Read the model definition and answer for the solid it produces. Units are mm, in the model's axes. Face numbers are marked on the shaded views. A direction names the side the tool comes from. Coordinates: 2 decimals unless noted, no trailing zeros. Write each loop counter-clockwise with the first axis right and the second up, starting at its lowest first coordinate (ties: lowest second). Pieces come first, ordered by that corner, then holes.
(1) The mould has two halves that part along Z. Classify the marked faces 4, 5 and 6: +Z half, -Z half, draft (parallel to the pull), parting line (faces both ways), or undercut.
(2) Section A-A on x = 36 is taken. Write down the section's boundary in (y, z), then the cut area to 3 significant figures.
(3) Find the intervals of material crossed by probe 1 along Z at (x, y) = (-65.5, -1); probe 2 along Z at (x, y) = (50, -6.5); probe 3 along Z at (x, y) = (19.5, 4.5), in increasing order.
(4) Which of the six approach directions +Z, -Z, +X, -X, +Y, -Y give full straight-line access (tool end or side, diameter ignored) to the marked faces 1, 2 and 3?
(5) Section B-B on y = 5.5 is taken. Write down the section's boundary in (x, z) (3 decimals), then the cut area to 3 significant figures.
(6) Section D-D on y = 32.5 is taken. Write down the section's boundary in (x, z), then the cut area to 3 significant figures.
(7) Section C-C on z = 0 is taken. Write down the section's boundary in (x, y) (3 decimals).
(8) Given pin 1 (22 mm diameter, centred on x = 32, z = -50, fed in from +Y); pin 2 (15 mm diameter, centred on x = -6, y = 13.5, fed in from +Z), each flat-ended and moving along its own axis, determine where each tip first touches the part or whether it passes through.
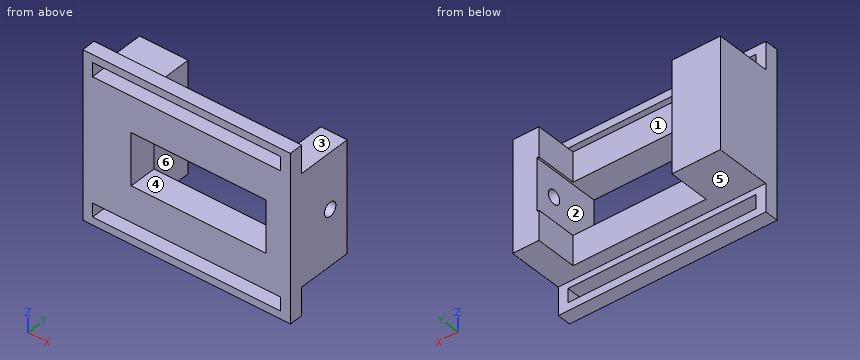
from build123d import *

# Parameters (mm, degrees)
SKETCH_1_W          = 150
SKETCH_1_H          = 80
EXTRUDE_1_DEPTH     = 40
SKETCH_2_W          = 150
SKETCH_2_H          = 120
SKETCH_2_W_2        = 135.983002124
SKETCH_2_H_2        = 10
EXTRUDE_2_DEPTH     = 10
SKETCH_3_W          = 96.092988376
SKETCH_3_H          = 30
CUT_EXTRUDE_1_DEPTH = 101
SKETCH_5_W          = 97.510223457
SKETCH_5_H          = 37.534840072
CUT_EXTRUDE_2_DEPTH = 51
SKETCH_6_R          = 5
CUT_EXTRUDE_3_DEPTH = 30


with BuildPart() as part:
    # Эскиз1 → Бобышка-Вытянуть1 (new body)
    with BuildSketch(Plane(origin=(0, 0, 0), x_dir=(1, 0, 0), z_dir=(0, 1, 0))):
        Rectangle(SKETCH_1_W, SKETCH_1_H)
    extrude(amount=EXTRUDE_1_DEPTH)

    # Эскиз2 → Бобышка-Вытянуть2 (add)
    with BuildSketch(Plane.XZ):
        Rectangle(SKETCH_2_W, SKETCH_2_H)
        with Locations((0, 49.39320085)):
            Rectangle(SKETCH_2_W_2, SKETCH_2_H_2, mode=Mode.SUBTRACT)
        with Locations((0, -49.39320085)):
            Rectangle(SKETCH_2_W_2, SKETCH_2_H_2, mode=Mode.SUBTRACT)
    extrude(amount=EXTRUDE_2_DEPTH)

    # Эскиз3 → Вырез-Вытянуть1 (cut, through all)
    with BuildSketch(Plane.XY.offset(40)):
        with Locations((8.046494188, 25)):
            Rectangle(SKETCH_3_W, SKETCH_3_H)
    extrude(amount=-CUT_EXTRUDE_1_DEPTH, mode=Mode.SUBTRACT)

    # Эскиз5 → Вырез-Вытянуть2 (cut, through all)
    with BuildSketch(Plane.XZ.offset(10)):
        with Locations((8.760111104, 0)):
            Rectangle(SKETCH_5_W, SKETCH_5_H)
    extrude(amount=-CUT_EXTRUDE_2_DEPTH, mode=Mode.SUBTRACT)

    # Эскиз6 → Вырез-Вытянуть3 (cut)
    with BuildSketch(Plane(origin=(75, 0, 0), x_dir=(0, 0, -1), z_dir=(1, 0, 0))):
        with Locations((0, 25)):
            Circle(SKETCH_6_R)
    extrude(amount=-CUT_EXTRUDE_3_DEPTH, mode=Mode.SUBTRACT)


solid = part.part
Response:
1. face 4: undercut
1. face 5: -Z half
1. face 6: draft
2. outline: (-10, -60) - (0, -60) - (0, -54.39) - (-10, -54.39) - close; (-10, -44.39) - (0, -44.39) - (0, -40) - (10, -40) - (10, -18.77) - (-10, -18.77) - close; (-10, 18.77) - (10, 18.77) - (10, 40) - (0, 40) - (0, 44.39) - (-10, 44.39) - close; (-10, 54.39) - (0, 54.39) - (0, 60) - (-10, 60) - close
2. area: 1,050 mm2
3. probe 1: z = -60 to -54.39, -44.39 to 44.39, 54.39 to 60
3. probe 2: z = -60 to -54.39, -44.39 to -18.77, 18.77 to 44.39, 54.39 to 60
3. probe 3: z = -40 to -18.77, 18.77 to 40
4. face 1: +Z, -Z, +Y
4. face 2: +Y, -Y
4. face 3: +Z, +X, -X, +Y
5. outline: (-75, -40) - (75, -40) - (75, 40) - (-75, 40) - close; hole (-39.995, -18.767) - (57.515, -18.767) - (57.515, 18.767) - (-39.995, 18.767) - close
5. area: 8,340 mm2
6. outline: (-75, -40) - (-40, -40) - (-40, 40) - (-75, 40) - close; (56.09, -40) - (75, -40) - (75, 40) - (56.09, 40) - (56.09, 18.77) - (57.52, 18.77) - (57.52, -18.77) - (56.09, -18.77) - close
6. area: 4,260 mm2
7. outline: (-75, -10) - (-39.995, -10) - (-39.995, 10) - (-40, 10) - (-40, 40) - (-75, 40) - close; (57.515, -10) - (75, -10) - (75, 20) - (57.515, 20) - close; (57.515, 30) - (75, 30) - (75, 40) - (57.515, 40) - close
8. pin 1: stops at y = 10
8. pin 2: stops at z = 40
